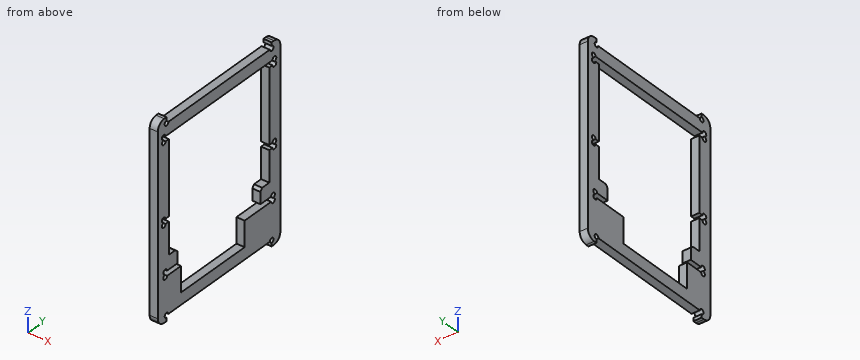
```python
from build123d import *

# Parameters (mm, degrees)
BOSS_EXTRUDE1_DEPTH = 5
FILLET1_R           = 5
CUT_EXTRUDE1_REACH  = 7
SKETCH2_W           = 3
SKETCH2_H           = 4
CUT_EXTRUDE2_REACH  = 7
SKETCH3_R           = 1.45


with BuildPart() as part:
    # Sketch1 → Boss-Extrude1 (new body)
    with BuildSketch(Plane(origin=(0, 0, 0), x_dir=(0, 0, -1), z_dir=(1, 0, 0))):
        Polygon((-59.36916415, -47.818646587), (0, -47.818646587), (59.36916415, -47.818646587), (59.36916415, -41), (55.86916415, -41), (55.86916415, 41), (59.36916415, 41), (59.36916415, 47.818646587), (-59.36916415, 47.818646587), (-59.36916415, 41), (-55.86916415, 41), (-55.86916415, -41), (-59.36916415, -41), align=None)
        Polygon((21.702610628, -39.175443067), (21.702610628, -34.307045578), (23.024909313, -32.569779859), (30.179141539, -32.569779859), (30.179141539, -42.076978078), (33.179141539, -42.076978078), (33.179141539, -29.710380013), (48.63820865, -29.710380013), (48.63820865, 19.945173818), (33.179141539, 19.945173818), (33.179141539, 42.076978078), (30.179141539, 42.076978078), (30.179141539, 32.288188968), (23.024909313, 32.288188968), (21.287643594, 33.610487654), (21.287643594, 39.175443067), (-48.63820865, 39.175443067), (-48.63820865, -39.175443067), align=None, mode=Mode.SUBTRACT)
    extrude(amount=BOSS_EXTRUDE1_DEPTH)

    # Fillet1
    fillet1_edges = [part.edges().sort_by_distance(p)[0] for p in [
        (2.5, -47.818646587, -59.36916415),
        (2.5, -47.818646587, 59.36916415),
        (2.5, 47.818646587, 59.36916415),
        (2.5, 47.818646587, -59.36916415),
    ]]
    fillet(fillet1_edges, radius=FILLET1_R)

    # Sketch2 → Cut-Extrude1 (cut, up to next)
    with BuildSketch(Plane.ZY, mode=Mode.PRIVATE) as cut_extrude1_sk1:
        with Locations((47.13820865, 41.175443067)):
            Rectangle(SKETCH2_W, SKETCH2_H)
    cut_extrude1_tool1 = extrude(cut_extrude1_sk1.sketch, amount=-CUT_EXTRUDE1_REACH, mode=Mode.PRIVATE) & part.part
    add(cut_extrude1_tool1.solids().sort_by_distance((0, 41.175443, 47.138209))[0], mode=Mode.SUBTRACT)
    # Sketch2 → Cut-Extrude1 (cut, up to next)
    with BuildSketch(Plane.ZY, mode=Mode.PRIVATE) as cut_extrude1_sk2:
        with Locations((47.13820865, -41.175443067)):
            Rectangle(SKETCH2_W, SKETCH2_H)
    cut_extrude1_tool2 = extrude(cut_extrude1_sk2.sketch, amount=-CUT_EXTRUDE1_REACH, mode=Mode.PRIVATE) & part.part
    add(cut_extrude1_tool2.solids().sort_by_distance((0, -41.175443, 47.138209))[0], mode=Mode.SUBTRACT)
    # Sketch2 → Cut-Extrude1 (cut, up to next)
    with BuildSketch(Plane.ZY, mode=Mode.PRIVATE) as cut_extrude1_sk3:
        with Locations((-0.884341096, -41.175443067)):
            Rectangle(SKETCH2_W, SKETCH2_H)
    cut_extrude1_tool3 = extrude(cut_extrude1_sk3.sketch, amount=-CUT_EXTRUDE1_REACH, mode=Mode.PRIVATE) & part.part
    add(cut_extrude1_tool3.solids().sort_by_distance((0, -41.175443, -0.884341))[0], mode=Mode.SUBTRACT)
    # Sketch2 → Cut-Extrude1 (cut, up to next)
    with BuildSketch(Plane.ZY, mode=Mode.PRIVATE) as cut_extrude1_sk4:
        with Locations((-0.884341096, 41.175443067)):
            Rectangle(SKETCH2_W, SKETCH2_H)
    cut_extrude1_tool4 = extrude(cut_extrude1_sk4.sketch, amount=-CUT_EXTRUDE1_REACH, mode=Mode.PRIVATE) & part.part
    add(cut_extrude1_tool4.solids().sort_by_distance((0, 41.175443, -0.884341))[0], mode=Mode.SUBTRACT)

    # Sketch3 → Cut-Extrude2 (cut, up to next)
    with BuildSketch(Plane.ZY, mode=Mode.PRIVATE) as cut_extrude2_sk1:
        with Locations((-33.179141539, 42.076978078)):
            Circle(SKETCH3_R)
    cut_extrude2_tool1 = extrude(cut_extrude2_sk1.sketch, amount=-CUT_EXTRUDE2_REACH, mode=Mode.PRIVATE) & part.part
    add(cut_extrude2_tool1.solids().sort_by_distance((0, 42.076978, -33.179142))[0], mode=Mode.SUBTRACT)
    # Sketch3 → Cut-Extrude2 (cut, up to next)
    with BuildSketch(Plane.ZY, mode=Mode.PRIVATE) as cut_extrude2_sk2:
        with Locations((-30.179141539, 42.076978078)):
            Circle(SKETCH3_R)
    cut_extrude2_tool2 = extrude(cut_extrude2_sk2.sketch, amount=-CUT_EXTRUDE2_REACH, mode=Mode.PRIVATE) & part.part
    add(cut_extrude2_tool2.solids().sort_by_distance((0, 42.076978, -30.179142))[0], mode=Mode.SUBTRACT)
    # Sketch3 → Cut-Extrude2 (cut, up to next)
    with BuildSketch(Plane.ZY, mode=Mode.PRIVATE) as cut_extrude2_sk3:
        with Locations((-2.384341096, 43.175443067)):
            Circle(SKETCH3_R)
    cut_extrude2_tool3 = extrude(cut_extrude2_sk3.sketch, amount=-CUT_EXTRUDE2_REACH, mode=Mode.PRIVATE) & part.part
    add(cut_extrude2_tool3.solids().sort_by_distance((0, 43.175443, -2.384341))[0], mode=Mode.SUBTRACT)
    # Sketch3 → Cut-Extrude2 (cut, up to next)
    with BuildSketch(Plane.ZY, mode=Mode.PRIVATE) as cut_extrude2_sk4:
        with Locations((0.615658904, 43.175443067)):
            Circle(SKETCH3_R)
    cut_extrude2_tool4 = extrude(cut_extrude2_sk4.sketch, amount=-CUT_EXTRUDE2_REACH, mode=Mode.PRIVATE) & part.part
    add(cut_extrude2_tool4.solids().sort_by_distance((0, 43.175443, 0.615659))[0], mode=Mode.SUBTRACT)
    # Sketch3 → Cut-Extrude2 (cut, up to next)
    with BuildSketch(Plane.ZY, mode=Mode.PRIVATE) as cut_extrude2_sk5:
        with Locations((-55.86916415, 41)):
            Circle(SKETCH3_R)
    cut_extrude2_tool5 = extrude(cut_extrude2_sk5.sketch, amount=-CUT_EXTRUDE2_REACH, mode=Mode.PRIVATE) & part.part
    add(cut_extrude2_tool5.solids().sort_by_distance((0, 41, -55.869164))[0], mode=Mode.SUBTRACT)
    # Sketch3 → Cut-Extrude2 (cut, up to next)
    with BuildSketch(Plane.ZY, mode=Mode.PRIVATE) as cut_extrude2_sk6:
        with Locations((45.63820865, 43.175443067)):
            Circle(SKETCH3_R)
    cut_extrude2_tool6 = extrude(cut_extrude2_sk6.sketch, amount=-CUT_EXTRUDE2_REACH, mode=Mode.PRIVATE) & part.part
    add(cut_extrude2_tool6.solids().sort_by_distance((0, 43.175443, 45.638209))[0], mode=Mode.SUBTRACT)
    # Sketch3 → Cut-Extrude2 (cut, up to next)
    with BuildSketch(Plane.ZY, mode=Mode.PRIVATE) as cut_extrude2_sk7:
        with Locations((48.63820865, 43.175443067)):
            Circle(SKETCH3_R)
    cut_extrude2_tool7 = extrude(cut_extrude2_sk7.sketch, amount=-CUT_EXTRUDE2_REACH, mode=Mode.PRIVATE) & part.part
    add(cut_extrude2_tool7.solids().sort_by_distance((0, 43.175443, 48.638209))[0], mode=Mode.SUBTRACT)
    # Sketch3 → Cut-Extrude2 (cut, up to next)
    with BuildSketch(Plane.ZY, mode=Mode.PRIVATE) as cut_extrude2_sk8:
        with Locations((48.63820865, -43.175443067)):
            Circle(SKETCH3_R)
    cut_extrude2_tool8 = extrude(cut_extrude2_sk8.sketch, amount=-CUT_EXTRUDE2_REACH, mode=Mode.PRIVATE) & part.part
    add(cut_extrude2_tool8.solids().sort_by_distance((0, -43.175443, 48.638209))[0], mode=Mode.SUBTRACT)
    # Sketch3 → Cut-Extrude2 (cut, up to next)
    with BuildSketch(Plane.ZY, mode=Mode.PRIVATE) as cut_extrude2_sk9:
        with Locations((45.63820865, -43.175443067)):
            Circle(SKETCH3_R)
    cut_extrude2_tool9 = extrude(cut_extrude2_sk9.sketch, amount=-CUT_EXTRUDE2_REACH, mode=Mode.PRIVATE) & part.part
    add(cut_extrude2_tool9.solids().sort_by_distance((0, -43.175443, 45.638209))[0], mode=Mode.SUBTRACT)
    # Sketch3 → Cut-Extrude2 (cut, up to next)
    with BuildSketch(Plane.ZY, mode=Mode.PRIVATE) as cut_extrude2_sk10:
        with Locations((0.615658904, -43.175443067)):
            Circle(SKETCH3_R)
    cut_extrude2_tool10 = extrude(cut_extrude2_sk10.sketch, amount=-CUT_EXTRUDE2_REACH, mode=Mode.PRIVATE) & part.part
    add(cut_extrude2_tool10.solids().sort_by_distance((0, -43.175443, 0.615659))[0], mode=Mode.SUBTRACT)
    # Sketch3 → Cut-Extrude2 (cut, up to next)
    with BuildSketch(Plane.ZY, mode=Mode.PRIVATE) as cut_extrude2_sk11:
        with Locations((-2.384341096, -43.175443067)):
            Circle(SKETCH3_R)
    cut_extrude2_tool11 = extrude(cut_extrude2_sk11.sketch, amount=-CUT_EXTRUDE2_REACH, mode=Mode.PRIVATE) & part.part
    add(cut_extrude2_tool11.solids().sort_by_distance((0, -43.175443, -2.384341))[0], mode=Mode.SUBTRACT)
    # Sketch3 → Cut-Extrude2 (cut, up to next)
    with BuildSketch(Plane.ZY, mode=Mode.PRIVATE) as cut_extrude2_sk12:
        with Locations((-30.179141539, -42.076978078)):
            Circle(SKETCH3_R)
    cut_extrude2_tool12 = extrude(cut_extrude2_sk12.sketch, amount=-CUT_EXTRUDE2_REACH, mode=Mode.PRIVATE) & part.part
    add(cut_extrude2_tool12.solids().sort_by_distance((0, -42.076978, -30.179142))[0], mode=Mode.SUBTRACT)
    # Sketch3 → Cut-Extrude2 (cut, up to next)
    with BuildSketch(Plane.ZY, mode=Mode.PRIVATE) as cut_extrude2_sk13:
        with Locations((-33.179141539, -42.076978078)):
            Circle(SKETCH3_R)
    cut_extrude2_tool13 = extrude(cut_extrude2_sk13.sketch, amount=-CUT_EXTRUDE2_REACH, mode=Mode.PRIVATE) & part.part
    add(cut_extrude2_tool13.solids().sort_by_distance((0, -42.076978, -33.179142))[0], mode=Mode.SUBTRACT)
    # Sketch3 → Cut-Extrude2 (cut, up to next)
    with BuildSketch(Plane.ZY, mode=Mode.PRIVATE) as cut_extrude2_sk14:
        with Locations((-55.86916415, -41)):
            Circle(SKETCH3_R)
    cut_extrude2_tool14 = extrude(cut_extrude2_sk14.sketch, amount=-CUT_EXTRUDE2_REACH, mode=Mode.PRIVATE) & part.part
    add(cut_extrude2_tool14.solids().sort_by_distance((0, -41, -55.869164))[0], mode=Mode.SUBTRACT)
    # Sketch3 → Cut-Extrude2 (cut, up to next)
    with BuildSketch(Plane.ZY, mode=Mode.PRIVATE) as cut_extrude2_sk15:
        with Locations((55.86916415, -41)):
            Circle(SKETCH3_R)
    cut_extrude2_tool15 = extrude(cut_extrude2_sk15.sketch, amount=-CUT_EXTRUDE2_REACH, mode=Mode.PRIVATE) & part.part
    add(cut_extrude2_tool15.solids().sort_by_distance((0, -41, 55.869164))[0], mode=Mode.SUBTRACT)
    # Sketch3 → Cut-Extrude2 (cut, up to next)
    with BuildSketch(Plane.ZY, mode=Mode.PRIVATE) as cut_extrude2_sk16:
        with Locations((55.86916415, 41)):
            Circle(SKETCH3_R)
    cut_extrude2_tool16 = extrude(cut_extrude2_sk16.sketch, amount=-CUT_EXTRUDE2_REACH, mode=Mode.PRIVATE) & part.part
    add(cut_extrude2_tool16.solids().sort_by_distance((0, 41, 55.869164))[0], mode=Mode.SUBTRACT)


solid = part.part
```
Design review of the part built by this model. Coordinates are the model's own, in mm. Give positions to 0.01 mm unless a question says otherwise; leave off trailing zeros. Loops run counter-clockwise (first coordinate to the right, second up) from the corner with the lowest first, then second, coordinate; pieces in that order, holes last. Notation, with made-up numbers: M 34,15.5 L 63,15.5 A34 ccw 63,49.5 Z; hole C 10,11 d2. An arc over 180 degrees is marked long. Return JSON: item names as keys, results as strings. Group by question number.
Item 1: Insertion check: pin 1 Ø2.5 at (x, z) = (3, 58) entering from +Y; pin 2 Ø1.5 at (x, y) = (4, -28.5) entering from +Z; pin 3 Ø1.5 at (x, y) = (1.5, -7) entering from -Z. Each pin has a flat end and moves straight along its axis. Give the tip position at first contact, or say it passes through.
Item 2: For probe 1 along Z at (x, y) = (2.3, -35.5); probe 2 along Z at (x, y) = (4.8, 34); probe 3 along Z at (x, y) = (4.05, 39.5), list the stretches that pass through material, from the lowest coordinate up.
Item 3: We need section B-B (z = -5.5). Give the boundary of the cut face in (x, y).
Item 4: We need section A-A (y = 9). Give the boundary of the cut face in (x, z).
Output:
{
 "1": {"pin 1": "stops at y = 47.22", "pin 2": "stops at z = 55.87", "pin 3": "stops at z = -55.87"},
 "2": {"probe 1": "z = -55.87 to -33.18, -30.18 to -21.7, 48.64 to 55.87", "probe 2": "z = -55.87 to -33.18, -30.18 to -21.29, 48.64 to 55.87", "probe 3": "z = -55.87 to -33.18, -30.18 to -2.38, 0.62 to 45.64, 48.64 to 55.87"},
 "3": {"outline": "M 0,-47.82 L 5,-47.82 L 5,-39.18 L 0,-39.18 Z; M 0,39.18 L 5,39.18 L 5,47.82 L 0,47.82 Z"},
 "4": {"outline": "M 0,-55.87 L 5,-55.87 L 5,-48.64 L 0,-48.64 Z; M 0,48.64 L 5,48.64 L 5,55.87 L 0,55.87 Z"}
}
